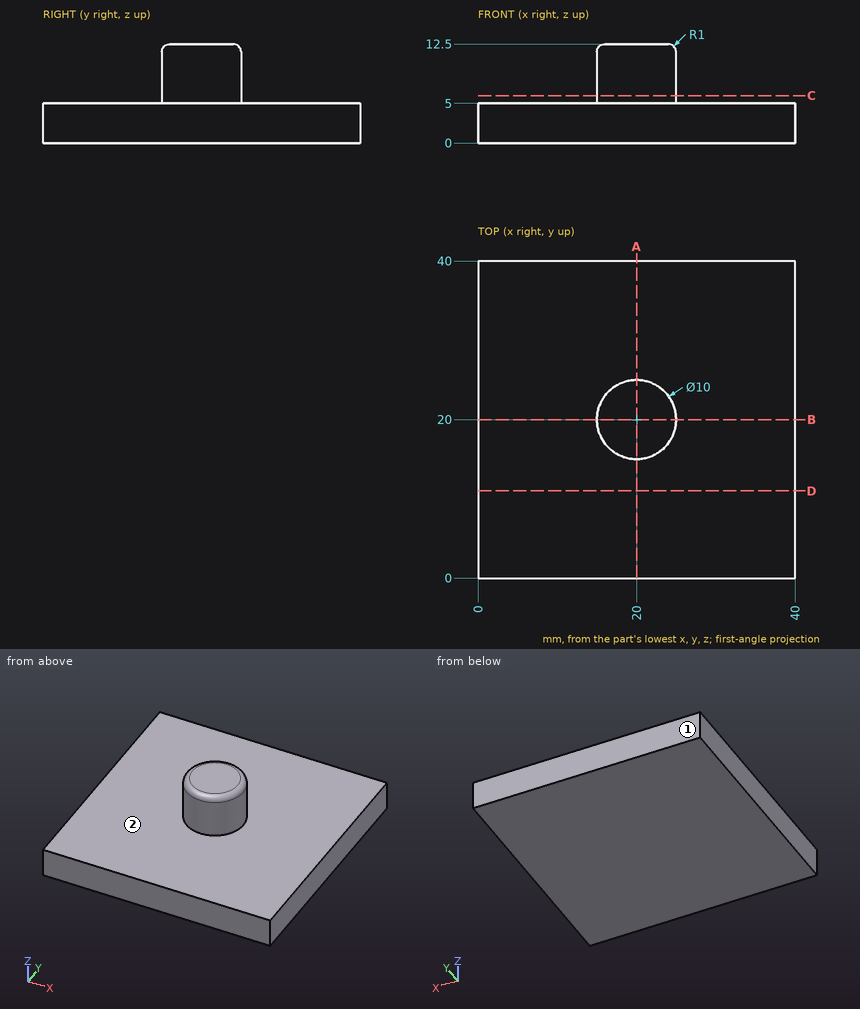
Design review of the part shown in the three views and the two pictorial views. Dimensions are in mm from the part's minimum x, y and z. A direction names the side the tool comes from. Give positions to 0.01 mm unless a question says otherwise; leave off trailing zeros. Loops run counter-clockwise (first coordinate to the right, second up) from the corner with the lowest first, then second, coordinate; pieces in that order, holes last. Notation, with made-up numbers: M 55.25,47.5 L 67.25,47.5 A12 cw 67.25,51.5 Z; hole C 41,14.25 d6. An arc over 180 degrees is marked long. Write item = value, one per line.
Q1. To check wall thickness, follow line 1 (Z direction, x = 23, y = 10); line 2 (X direction, y = 22.5, z = 7); line 3 (Y direction, x = 18, z = 9). State the ranges of each line that lie inside material, in increasing order. Write a range as [from, to].
Output values:
line_1 = [0, 5]
line_2 = [15.67, 24.33]
line_3 = [15.42, 24.58]
Q2. We need section D-D (y = 11). Give the boundary of the cut face in (x, z).
Output values:
outline = M 0,0 L 40,0 L 40,5 L 0,5 Z
Q3. We need section C-C (z = 6). Give the boundary of the cut face in (x, y), plus the area to 3 significant figures.
Output values:
outline = C 20,20 d10
area = 78.5 mm^2
Q4. We need section A-A (x = 20). Give the boundary of the cut face in (y, z).
Output values:
outline = M 0,0 L 40,0 L 40,5 L 25,5 L 25,11.5 A1 ccw 24,12.5 L 16,12.5 A1 ccw 15,11.5 L 15,5 L 0,5 Z
Q5. For the marked faces 1 and 2, list the 3-axis set-ups (+Z, -Z, +X, -X, +Y, -Y) from which the entire face can be reached by the end or side of a thin tool; tool diameter is ignored.
Output values:
face_1 = +Z, -Z, +X, -X, +Y
face_2 = +Z
Q6. Insertion check: pin 1 (1 mm diameter, centred on x = 33, y = 30.5, fed in from +Z). The pin has a flat end and moves straight along its axis. Give the tip position at first contact, or say it passes through.
Output values:
pin_1 = 5
